Input: part model. Units: mm. Frame: model coordinates. Face numbers are marked on the shaded views. A direction names the side the tool comes from. Coordinates: 2 decimals unless noted, no trailing zeros. Write each loop counter-clockwise with the first axis right and the second up, starting at its lowest first coordinate (ties: lowest second). Pieces come first, ordered by that corner, then holes. Notation, with made-up numbers: (-33, 31.5) - (11, 31.5) arc R21 ccw to (11, 44.5) - close; hole circle Ø2 at (-19, -16.75). An arc over 180 degrees is marked (long way). Use a Markdown table: item, result. Add a question column.
Q1. Material intervals for probe 1 along Y at (x, z) = (0, 5.5); probe 2 along X at (y, z) = (-1.5, 9.5), sorted ascending. Write a range as from..to.
Q2. Section query D-D (y = -2.75). Return the cut outline in (x, z).
Q3. Section query A-A (x = 0). Return the cut outline in (y, z), then the cut area to 3 significant figures.
Q4. Mould query, pull axis X, two halves, no side actions, for the marked faces 1, 2 and 3. Classes: released by +X, released by -X, zero draft, split by the parting line, or undercut.
Q5. Set-up query: the marked faces 4 and 5. Return all of +Z, -Z, +X, -X, +Y, -Y with unobstructed straight access to the full face (end or side cutting, diameter ignored); none if empty.
Q6. Pin query (flat end, axial travel): P1, Ø3, axis at y = -3, z = 8, coming from the -X side; P2, Ø4, axis at x = 4, z = 2.5, coming from the +Y side; P3, Ø1, axis at y = -1, z = 5, coming from the +X side; P4, Ø0.9, axis at y = 1.5, z = 2, coming from the +X side. Return the tip coordinate at first contact, or that it passes through.
Q7. Section query C-C (y = 3). Return the cut outline in (x, z).
from build123d import *

# Parameters (mm, degrees)
F1_W     = 43
F1_H     = 7.7
F1_R     = 1.9
F3_DEPTH = 11.2
F2_R     = 3.4
F2_R_2   = 1.9
F4_DEPTH = 3
F5_R     = 3.84999
F6_W     = 8.2597071305
F6_H     = 7.7
F6_H_2   = 7.1181999311
F7_DEPTH = 3


# Not quite as in the source:
# - a fillet or chamfer is up to 0.001 mm smaller than in the source, because OpenCascade refuses the exact size


with BuildPart() as f3:
    # F1 (on face) → F3 (new body)
    with BuildSketch(Plane.XY):
        Rectangle(F1_W, F1_H)
        Circle(F1_R, mode=Mode.SUBTRACT)
    extrude(amount=F3_DEPTH)

    # F2 (on face) → F4 (cut)
    with BuildSketch(Plane.XY):
        Circle(F2_R)
        Circle(F2_R_2, mode=Mode.SUBTRACT)
    extrude(amount=F4_DEPTH, mode=Mode.SUBTRACT)

    # F5 (radius 3.85 in the source; OpenCascade refuses exactly that, so slightly less here)
    f5_edges = [f3.edges().sort_by_distance(p)[0] for p in [
        (-21.5, -3.85, 5.6),
        (-21.5, 3.85, 5.6),
        (21.5, -3.85, 5.6),
        (21.5, 3.85, 5.6),
    ]]
    fillet(f5_edges, radius=F5_R)

    # F6 (on face) → F7 (cut)
    with BuildSketch(Plane.XY):
        Rectangle(F6_W, F6_H)
        with Locations((0, -7.4090999655)):
            Rectangle(F6_W, F6_H_2)
        with Locations((0, 7.4090999655)):
            Rectangle(F6_W, F6_H_2)
    extrude(amount=F7_DEPTH, mode=Mode.SUBTRACT)


solid = f3.part
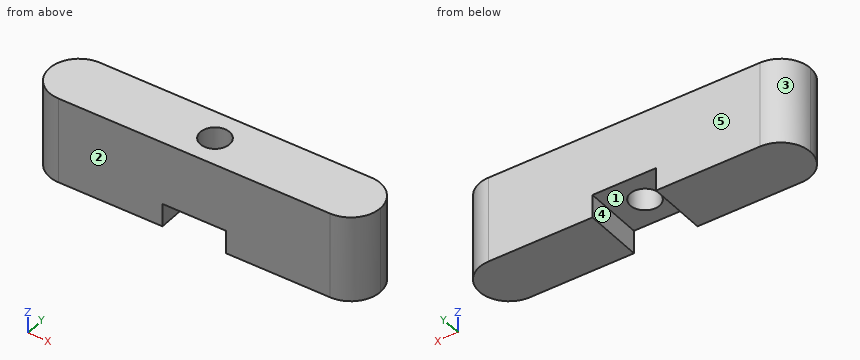
Values follow:
| question | item | result |
|---|---|---|
| 1 | probe 1 | -3.85..-1.9, 1.9..3.85 |
| 1 | probe 2 | -21.2..-1.17, 1.17..21.2 |
| 2 | outline | (-20.34, 0) - (-4.13, 0) - (-4.13, 3) - (4.13, 3) - (4.13, 0) - (20.34, 0) - (20.34, 11.2) - (-20.34, 11.2) - close |
| 3 | outline | (-3.85, 3) - (-1.9, 3) - (-1.9, 11.2) - (-3.85, 11.2) - close; (1.9, 3) - (3.85, 3) - (3.85, 11.2) - (1.9, 11.2) - close |
| 3 | area | 32.0 mm2 |
| 4 | face 1 | undercut |
| 4 | face 2 | zero draft |
| 4 | face 3 | released by -X |
| 5 | face 4 | -Z, +Y, -Y |
| 5 | face 5 | +Z, -Z, +X, -X, +Y |
| 6 | P1 | x = -21.2 |
| 6 | P2 | y = 3.85 |
| 6 | P3 | x = 21.47 |
| 6 | P4 | x = 21.35 |
| 7 | outline | (-20.06, 0) - (-4.13, 0) - (-4.13, 3) - (4.13, 3) - (4.13, 0) - (20.06, 0) - (20.06, 11.2) - (-20.06, 11.2) - close |
